```python
from build123d import *

# Parameters (mm, degrees)
BOX001_W               = 10
BOX001_H               = 2
BOX001_DEPTH           = 2
BOX001_PLACEMENT_ANGLE = 20
BOX_W                  = 10
BOX_H                  = 2
BOX_DEPTH              = 2
BOX_PLACEMENT_ANGLE    = 20
FUSION_PLACEMENT_ANGLE = 64


with BuildPart() as cube001:
    # Box001 → Box001 (new body)
    with BuildSketch(Plane.XY):
        with Locations((5, 1)):
            Rectangle(BOX001_W, BOX001_H)
    extrude(amount=BOX001_DEPTH)


with BuildPart() as cube001_1:
    # Box001 placement: moved
    add(cube001.part.moved(Location((-5.040483, 0.770408, 0))).rotate(Axis((-5.040483, 0.770408, 0), (0, 0, -1)), BOX001_PLACEMENT_ANGLE))


with BuildPart() as fusion:
    # Box → Box (new body)
    with BuildSketch(Plane.XY):
        with Locations((5, 1)):
            Rectangle(BOX_W, BOX_H)
    extrude(amount=BOX_DEPTH)


with BuildPart() as fusion_1:
    # Box placement: moved
    add(fusion.part.moved(Location((-4.356443, -2.649793, 0))).rotate(Axis((-4.356443, -2.649793, 0), (0, 0, 1)), BOX_PLACEMENT_ANGLE))

    # Fusion: union Cube001
    add(cube001_1.part)


with BuildPart() as fusion_2:
    # Fusion placement: moved
    add(fusion_1.part.rotate(Axis((0, 0, 0), (0, 0, 1)), FUSION_PLACEMENT_ANGLE))


solid = fusion_2.part
```
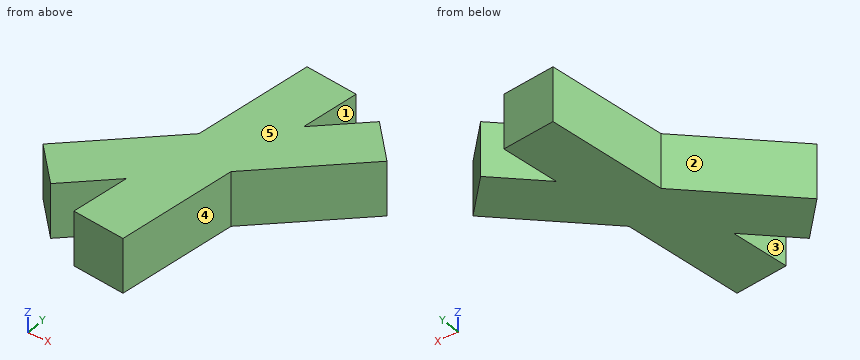
Build history of the part. All positions in model axes, mm. Face numbers are marked on the shaded views. A direction names the side the tool comes from. Give positions to 0.01 mm unless a question says otherwise; leave off trailing zeros. Loops run counter-clockwise (first coordinate to the right, second up) from the corner with the lowest first, then second, coordinate; pieces in that order, holes last.
Item 1: Pull direction X, two halves, no side cores. Call the marked faces 3, 4 and 5: released by +X, released by -X, zero draft, split by the parting line, or undercut.
Answers follow:
face 3: undercut
face 4: released by +X
face 5: zero draft
Item 2: Slice it at D-D, the plane y = -0.75. List the corners of the cut face in (x, z).
Answers follow:
outline: (-2.22, 0) - (0.93, 0) - (0.93, 2) - (-2.22, 2) - close
Item 3: Which spindle directions (+Z, -Z, +X, -X, +Y, -Y) get a long thin tool onto all of the face, cutting with end or side? Do the marked faces 1 and 2. Say none if no direction does.
Answers follow:
face 1: +Z, -Z
face 2: +Z, -Z, -X, +Y
Item 4: Slice it at A-A, the plane z = 0.55. List the corners of the cut face in (x, y).
Answers follow:
outline: (-4.29, -2.75) - (-2.9, -4.19) - (-1.28, -2.63) - (-1.52, -4.87) - (0.47, -5.08) - (0.96, -0.47) - (4.29, 2.75) - (2.9, 4.19) - (1.28, 2.63) - (1.52, 4.87) - (-0.47, 5.08) - (-0.96, 0.47) - close
Item 5: Slice it at B-B, the plane y = -3. List the corners of the cut face in (x, z).
Answers follow:
outline: (-4.05, 0) - (-1.67, 0) - (-1.67, 2) - (-4.05, 2) - close; (-1.32, 0) - (0.69, 0) - (0.69, 2) - (-1.32, 2) - close
Item 6: Drill centre lines: line 1 (X direction, y = -4, z = 0.5); line 2 (X direction, y = -3.25, z = 0.1); line 3 (X direction, y = -0.5, z = 1.05). Where is each one in solid material? Low to high.
Answers follow:
line 1: x = -3.09 to -2.7, -1.43 to 0.59
line 2: x = -3.81 to -1.93, -1.35 to 0.66
line 3: x = -1.96 to 0.95
Item 7: Slice it at C-C, the plane y = 2.5. List the corners of the cut face in (x, z).
Answers follow:
outline: (-0.74, 0) - (4.03, 0) - (4.03, 2) - (-0.74, 2) - close
